Part model, mm, in its own coordinate system. Face numbers are marked on the shaded views. A direction names the side the tool comes from. Give positions to 0.01 mm unless a question says otherwise; leave off trailing zeros. Order: outer loops, then holes, each group sorted by start corner. A loop starts at its lowest first (then second) coordinate and runs counter-clockwise, first axis right, second up. Notation, with made-up numbers: (47, 71.25) - (71, 71.25) arc R20 ccw to (71, 107.25) - close; hole circle Ø2 at (-17, -11). An arc over 180 degrees is marked (long way). Use a Markdown table: item, result. Add a question column.
from build123d import *

# Parameters (mm, degrees)
F0_W      = 69.85
F0_H      = 44.45
F1_DEPTH  = 12.7
F2_T      = -6.35
F3_R      = 3.81
F4_R      = 2.54
F5_R      = 1.5875
F5_R_2    = 1.905
F6_DEPTH  = 5.08
F7_R      = 2.8575
F8_DEPTH  = 12.446
F9_R      = 2.54
F10_DEPTH = 6.35
F12_DEPTH = 3.175


# Not quite as in the source:
# - a feature names something its author has since deleted; it is built from what else it names


with BuildPart() as f1:
    # F0 (on Front) → F1 (new body)
    with BuildSketch(Plane.XZ):
        Rectangle(F0_W, F0_H)
    extrude(amount=-F1_DEPTH)

    # F2
    f2_openings = [f1.faces().sort_by_distance(p)[0] for p in [
        (0, 0, 0),
    ]]
    offset(amount=F2_T, openings=f2_openings)

    # F3
    f3_edges = [f1.edges().sort_by_distance(p)[0] for p in [
        (34.925, 6.35, -22.225),
        (34.925, 12.7, 0),
        (0, 12.7, -22.225),
        (-34.925, 12.7, 0),
        (0, 12.7, 22.225),
        (-34.925, 6.35, 22.225),
        (34.925, 6.35, 22.225),
        (-34.925, 6.35, -22.225),
    ]]
    fillet(f3_edges, radius=F3_R)

    # F4
    f4_edges = [f1.edges().sort_by_distance(p)[0] for p in [
        (-28.575, 6.35, 0),
        (0, 6.35, -15.875),
        (28.575, 6.35, 0),
        (0, 6.35, 15.875),
        (-28.575, 3.175, -15.875),
        (28.575, 3.175, -15.875),
        (28.575, 3.175, 15.875),
        (-28.575, 3.175, 15.875),
    ]]
    fillet(f4_edges, radius=F4_R)

    # F5 (on face) → F6 (cut)
    with BuildSketch(Plane.XZ):
        with Locations((-31.115, 18.415)):
            Circle(F5_R)
        with Locations((31.115, -18.415)):
            Circle(F5_R_2)
    extrude(amount=-F6_DEPTH, mode=Mode.SUBTRACT)

    # F7 (on face) → F8 (join)
    with BuildSketch(Plane.XZ.offset(-6.35)):
        with Locations((-14.605, 0)):
            Circle(F7_R)
        with Locations((12.065, 0)):
            Circle(F7_R)
    extrude(amount=F8_DEPTH)

    # F9 (on face) → F10 (cut, through all)
    with BuildSketch(Plane.XY.offset(22.225)):
        with Locations((-5.08, 0)):
            Circle(F9_R)
        with Locations((21.59, 0)):
            Circle(F9_R)
    extrude(amount=-F10_DEPTH, mode=Mode.SUBTRACT)

    # F11 (on face) → F12 (cut)
    with BuildSketch(Plane(origin=(0, 0, 15.875), x_dir=(1, 0, 0), z_dir=(0, 0, -1))):
        with BuildLine():
            add(Edge.make_bspline(
                [(-8.89, 0), (-8.89, -1.6497783942), (-3.175, -0.8248891971), (2.54, 0), (-3.175, 0.8248891971), (-8.89, 1.6497783942), (-8.89, 0)],
                knots=[0, 0, 0, 2.0943951024, 2.0943951024, 4.1887902048, 4.1887902048, 6.2831853072, 6.2831853072, 6.2831853072], degree=2, weights=[1, 0.5, 1, 0.5, 1, 0.5, 1]))
        make_face()
        with BuildLine():
            add(Edge.make_bspline(
                [(17.78, 0), (17.78, -1.6497783942), (23.495, -0.8248891971), (29.21, 0), (23.495, 0.8248891971), (17.78, 1.6497783942), (17.78, 0)],
                knots=[0, 0, 0, 2.0943951024, 2.0943951024, 4.1887902048, 4.1887902048, 6.2831853072, 6.2831853072, 6.2831853072], degree=2, weights=[1, 0.5, 1, 0.5, 1, 0.5, 1]))
        make_face()
    extrude(amount=-F12_DEPTH, mode=Mode.SUBTRACT)


solid = f1.part
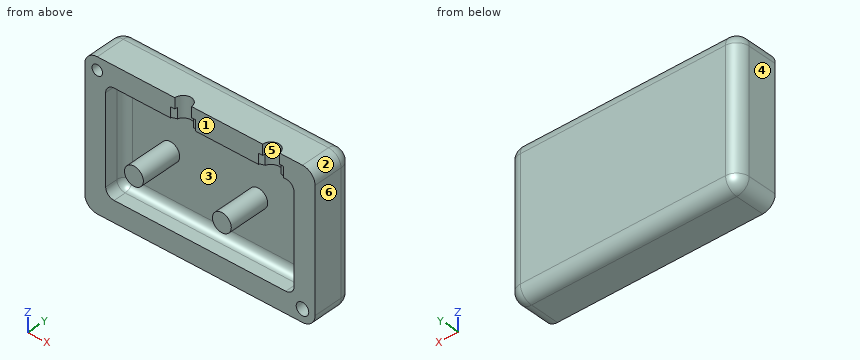
1. Cut at B-B (x = -21.5). Write the cut outline in (y, z) (3 decimals), plus the area to 3 significant figures.
2. Pin check, flat tips, straight feed: P1, Ø2.5, axis at x = -31.115, z = 18.415, coming from the -Y side; P2, Ø8, axis at x = 2.5, z = 6, coming from the -Y side; P3, Ø1.9, axis at x = 3.5, z = 17.5, coming from the -Y side; P4, Ø5, axis at y = -1, z = -13, coming from the -X side (3 decimals). Stop position of each tip, or through.
3. Tool access for the marked faces 1, 2 and 3: list every direction of +Z, -Z, +X, -X, +Y, -Y with a clear straight run to the whole face (end or side of a thin tool).
4. Mould opens along X. For the marked faces 4, 5 and 6 say: released by +X, released by -X, zero draft, split by the parting line, or undercut.
5. Cut at C-C (y = -1.5). Write the cut outline in (x, z) (1 decimal), plus the area to 3 significant figures.
6. Cut at D-D (y = 10.75). Write the cut outline in (x, z) (3 decimals).
7. Drill centre lines: probe 1 along X at (y, z) = (3.75, -4.5) (3 decimals); probe 2 along Y at (x, z) = (-15.5, -11.5); probe 3 along X at (y, z) = (9, -14). Where is each one in solid material? Low to high. Write a range as [from, to].
8. Cut at A-A (z = 8). Write the cut outline in (x, y) (3 decimals), plus the area to 3 significant figures.
Responses:
| question | item | result |
|---|---|---|
| 1 | outline | (0, -22.225) - (8.89, -22.225) arc R3.81 ccw to (12.7, -18.415) - (12.7, 18.415) arc R3.81 ccw to (8.89, 22.225) - (0, 22.225) - (0, 15.875) - (3.81, 15.875) arc R2.54 cw to (6.35, 13.335) - (6.35, -13.335) arc R2.54 cw to (3.81, -15.875) - (0, -15.875) - close |
| 1 | area | 359 mm² |
| 2 | P1 | stops at y = 5.08 |
| 2 | P2 | stops at y = 6.35 |
| 2 | P3 | stops at y = 0 |
| 2 | P4 | stops at x = -34.925 |
| 3 | face 1 | +Z, +X, -X, -Y |
| 3 | face 2 | +Z, +X, +Y, -Y |
| 3 | face 3 | -Y |
| 4 | face 4 | released by -X |
| 4 | face 5 | undercut |
| 4 | face 6 | released by +X |
| 5 | outline | circle Ø5.7 at (-14.6, 0); circle Ø5.7 at (12.1, 0) |
| 5 | area | 51.3 mm² |
| 6 | outline | (-34.44, -18.415) arc R3.325 ccw to (-31.115, -21.74) - (31.115, -21.74) arc R3.325 ccw to (34.44, -18.415) - (34.44, 18.415) arc R3.325 ccw to (31.115, 21.74) - (-31.115, 21.74) arc R3.325 ccw to (-34.44, 18.415) - close |
| 7 | probe 1 | x = [-34.925, -28.575], [28.575, 34.925] |
| 7 | probe 2 | y = [6.35, 12.7] |
| 7 | probe 3 | x = [-34.92, 34.92] |
| 8 | outline | (-34.925, 0) - (-28.575, 0) - (-28.575, 3.81) arc R2.54 cw to (-26.035, 6.35) - (26.035, 6.35) arc R2.54 cw to (28.575, 3.81) - (28.575, 0) - (34.925, 0) - (34.925, 8.89) arc R3.81 ccw to (31.115, 12.7) - (-31.115, 12.7) arc R3.81 ccw to (-34.925, 8.89) - close |
| 8 | area | 521 mm² |
